Can you work these out from the model? Positions are in its coordinate system, mm. Face numbers are marked on the shaded views. A direction names the side the tool comes from. Coordinates: 2 decimals unless noted, no trailing zeros. Loops run counter-clockwise (first coordinate to the right, second up) from the corner with the lowest first, then second, coordinate; pieces in that order, holes last. Notation, with made-up numbers: (40.25, 83) -> (48.25, 83) arc R9 cw to (48.25, 91) -> close; hole circle Ø1 at (63, 41). An arc over 180 degrees is marked (long way). Put each result on its own line as item: value. Start each with the question number.
Item 1: If we section it at A-A on x = 17.8: Please give me the cut outline in (y, z), plus the area to 3 significant figures.
Item 2: For the marked faces 3, 4, 5 and 6, which set-ups out of +Z, -Z, +X, -X, +Y, -Y let a thin tool reach every point of the face, with its end or its side?
Item 3: If we section it at B-B on y = 0: Please give me the cut outline in (x, z), plus the area to 3 significant figures.
Item 4: Will these pins go through, and if not, where does the flat tip stop? P1, Ø1, axis at x = 2, z = 6, coming from the +Y side; P2, Ø1.5, axis at y = 12, z = 1.5, coming from the -X side; P3, Ø14.5, axis at x = 11.5, y = -7.5, coming from the +Z side.
Item 5: We'd pull the mould along Y, two halves only. Please class the marked faces 1 and 2: pulls with the +Y half, pulls with the -Y half, needs draft (parallel to the pull), parting line crosses it, or undercut.
Item 6: Please list where these lines run through material, in increasing order: L1, parallel to Y at x = -8, z = 1.75; L2, parallel to X at y = 0, z = 1; L3, parallel to Y at x = -9, z = 4.25. Write a range as from..to.
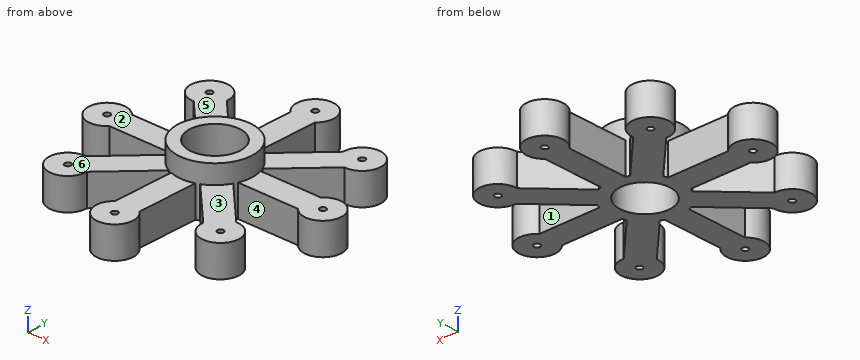
```python
from build123d import *

# Parameters (mm, degrees)
F1_R            = 6
F2_DEPTH        = 8
F0_R            = 0.5
F3_DEPTH        = 5
F3_COPIES_COUNT = 8
F4_R            = 4.1
F5_DEPTH        = 8.001


# Not quite as in the source:
# - a pattern or mirror of a feature is missing from the dataset's text; its kind, count and spacing are read off the source's solid


with BuildPart() as f2:
    # F1 (on Top) → F2 (new body)
    with BuildSketch(Plane.XY):
        Circle(F1_R)
    extrude(amount=F2_DEPTH)

    # F0 (on Top) → F3 (join)
    with BuildSketch(Plane.XY):
        with BuildLine():
            Line((0, 2), (-15.5639320225, 2))
            ThreePointArc((-15.5639320225, 2), (-20.8, 0), (-15.5639320225, -2))
            Line((-15.5639320225, -2), (0, -2))
            Line((0, -2), (0, 2))
        make_face()
        with Locations((-17.8, 0)):
            Circle(F0_R, mode=Mode.SUBTRACT)
    f3 = extrude(amount=F3_DEPTH)

    # F3_copies: F3 ×8 about axis
    f3_copies_axis = Axis((0, 0, 0), (0, 0, 1))
    for i in range(1, F3_COPIES_COUNT):
        add(f3.rotate(f3_copies_axis, i * 360 / F3_COPIES_COUNT))

    # F4 (on Top) → F5 (cut, through all)
    with BuildSketch(Plane.XY):
        Circle(F4_R)
    extrude(amount=F5_DEPTH, mode=Mode.SUBTRACT)


solid = f2.part
```
Solutions:
1. outline: (-3, 0) -> (-0.5, 0) -> (-0.5, 5) -> (-3, 5) -> close; (0.5, 0) -> (3, 0) -> (3, 5) -> (0.5, 5) -> close
1. area: 25.0 mm^2
2. face 3: +Z, +X, -Y
2. face 4: +Z, -Z
2. face 5: +Z, -X, +Y
2. face 6: +Z, -X, -Y
3. outline: (-20.8, 0) -> (-18.3, 0) -> (-18.3, 5) -> (-20.8, 5) -> close; (-17.3, 0) -> (-4.1, 0) -> (-4.1, 8) -> (-6, 8) -> (-6, 5) -> (-17.3, 5) -> close; (4.1, 0) -> (17.3, 0) -> (17.3, 5) -> (6, 5) -> (6, 8) -> (4.1, 8) -> close; (18.3, 0) -> (20.8, 0) -> (20.8, 5) -> (18.3, 5) -> close
3. area: 168 mm^2
4. P1: y = 5.81
4. P2: x = -15.59
4. P3: z = 5
5. face 1: undercut
5. face 2: needs draft
6. L1: -10.83..-5.17, -2..2, 5.17..10.83
6. L2: -20.8..-18.3, -17.3..-4.1, 4.1..17.3, 18.3..20.8
6. L3: -11.83..-6.17, -2..2, 6.17..11.83
